Read the model definition and answer for the solid it produces. Units are mm, in the model's axes. Coordinates: 2 decimals unless noted, no trailing zeros.
1) Each of these flat-tipped pins is pushed along its axis until it touches: pin 1 Ø6 at (x, y) = (-11.5, -5) entering from -Z; pin 2 Ø8 at (x, y) = (-31.5, -3) entering from -Z; pin 3 Ø6 at (y, z) = (-3.5, -4) entering from -X. Where does it stop, or does it pass through?
2) Find the intervals of material crossed by line 1 (Z direction, x = 0, y = -13); line 2 (Z direction, x = 2.5, y = -12.25); line 3 (Z direction, x = -36.5, y = -4), in increasing order.
3) Determine the mould class of faces 1 (the face through (-11.012, -9.413, -49.592)), 2 (the face through (21, -19.05, 1)), 3 (the face through (-13.858, -9.413, -10.626)) for opening direction X: +X half, -X half, draft (parallel to the pull), parting line (faces both ways), or undercut.
4) The part is cut by section A-A (x = 0). Give the number of separate pieces and of enclosed holes in the cut face, then the cut area to 3 significant figures.
from build123d import *

# Parameters (mm, degrees)
F0_R     = 50.8
F0_R_2   = 6.35
F0_R_3   = 17.4625
F1_DEPTH = 19.05
F2_SIZE  = 1.524
F3_SIZE  = 1.524
F4_SIZE  = 1.524
F5_SIZE  = 1.524
F6_SIZE  = 1.524
F7_SIZE  = 1.524
F8_SIZE  = 1.524
F9_SIZE  = 1.524


with BuildPart() as f1:
    # F0 (on Front) → F1 (new body)
    with BuildSketch(Plane.XZ):
        Circle(F0_R)
        with Locations((0, -33.3375)):
            Circle(F0_R_2, mode=Mode.SUBTRACT)
        with Locations((-33.3375, 0)):
            Circle(F0_R_2, mode=Mode.SUBTRACT)
        Circle(F0_R_3, mode=Mode.SUBTRACT)
        with Locations((33.3375, 0)):
            Circle(F0_R_2, mode=Mode.SUBTRACT)
        with Locations((0, 33.3375)):
            Circle(F0_R_2, mode=Mode.SUBTRACT)
    extrude(amount=F1_DEPTH)

    # F2
    f2_edges = [f1.edges().sort_by_distance(p)[0] for p in [
        (-50.8, -19.05, 0),
    ]]
    chamfer(f2_edges, length=F2_SIZE)

    # F3
    f3_edges = [f1.edges().sort_by_distance(p)[0] for p in [
        (-6.35, -19.05, 33.3375),
    ]]
    chamfer(f3_edges, length=F3_SIZE)

    # F4
    f4_edges = [f1.edges().sort_by_distance(p)[0] for p in [
        (-39.6875, -19.05, 0),
    ]]
    chamfer(f4_edges, length=F4_SIZE)

    # F5
    f5_edges = [f1.edges().sort_by_distance(p)[0] for p in [
        (-6.35, -19.05, -33.3375),
    ]]
    chamfer(f5_edges, length=F5_SIZE)

    # F6
    f6_edges = [f1.edges().sort_by_distance(p)[0] for p in [
        (26.9875, -19.05, 0),
    ]]
    chamfer(f6_edges, length=F6_SIZE)

    # F7
    f7_edges = [f1.edges().sort_by_distance(p)[0] for p in [
        (-17.4625, -19.05, 0),
    ]]
    chamfer(f7_edges, length=F7_SIZE)

    # F8
    f8_edges = [f1.edges().sort_by_distance(p)[0] for p in [
        (-50.8, 0, 0),
    ]]
    chamfer(f8_edges, length=F8_SIZE)

    # F9
    f9_edges = [f1.edges().sort_by_distance(p)[0] for p in [
        (-6.35, 0, -33.3375),
        (26.9875, 0, 0),
        (-6.35, 0, 33.3375),
        (-39.6875, 0, 0),
        (-17.4625, 0, 0),
    ]]
    chamfer(f9_edges, length=F9_SIZE)


solid = f1.part
Reported:
1. pin 1: stops at z = -50.08
1. pin 2: stops at z = -42.71
1. pin 3: stops at x = -50.79
2. line 1: z = -50.8 to -39.69, -26.99 to -17.46, 17.46 to 26.99, 39.69 to 50.8
2. line 2: z = -50.74 to -39.17, -27.5 to -17.28, 17.28 to 27.5, 39.17 to 50.74
2. line 3: z = -35.33 to -5.51, 5.51 to 35.33
3. face 1: parting line
3. face 2: draft
3. face 3: undercut
4. separate pieces: 4
4. enclosed holes: 0
4. area: 768 mm2
